Can you work these out from the drawing? Everything is in mm from the part's minimum corner. Round coordinates to 2 decimals unless told otherwise and drop trailing zeros. Order: outer loops, then holes, each group sorted by start corner. A loop starts at its lowest first (then second) coordinate and runs counter-clockwise, first axis right, second up. Notation, with made-up numbers: (12.25, -7) -> (39.25, -7) arc R34 ccw to (39.25, 30) -> close; hole circle Ø7 at (-13.75, 85). An arc over 180 degrees is marked (long way). One line per item, written item: value.
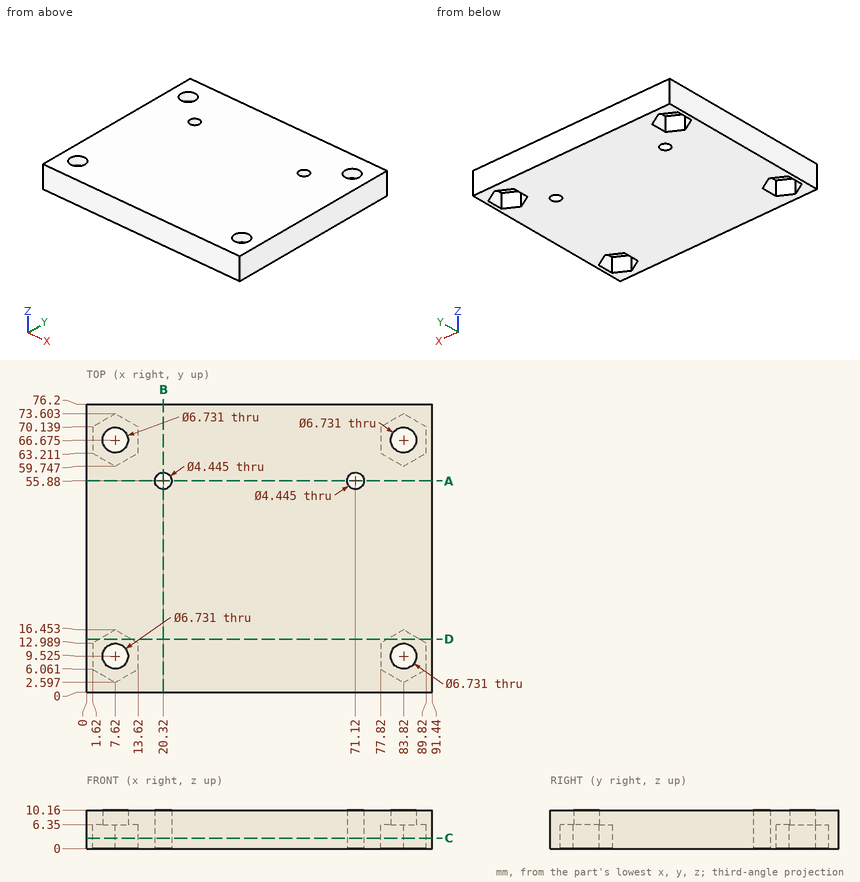
Q1. I want a section at D-D on y = 14. Write out the boundary of the cut face in (x, z), then the cut area to 3 significant figures.
Answers:
outline: (0, 0) -> (3.37, 0) -> (3.37, 6.35) -> (11.87, 6.35) -> (11.87, 0) -> (79.57, 0) -> (79.57, 6.35) -> (88.07, 6.35) -> (88.07, 0) -> (91.44, 0) -> (91.44, 10.16) -> (0, 10.16) -> close
area: 821 mm2
Q2. I want a section at A-A on y = 55.88. Write out the boundary of the cut face in (x, z).
Answers:
outline: (0, 0) -> (18.1, 0) -> (18.1, 10.16) -> (0, 10.16) -> close; (22.54, 0) -> (68.9, 0) -> (68.9, 10.16) -> (22.54, 10.16) -> close; (73.34, 0) -> (91.44, 0) -> (91.44, 10.16) -> (73.34, 10.16) -> close
Q3. I want a section at B-B on x = 20.32. Write out the boundary of the cut face in (y, z), then the cut area to 3 significant figures.
Answers:
outline: (0, 0) -> (53.66, 0) -> (53.66, 10.16) -> (0, 10.16) -> close; (58.1, 0) -> (76.2, 0) -> (76.2, 10.16) -> (58.1, 10.16) -> close
area: 729 mm2
Q4. I need wall thicknesses on line 1 along X through (y, z) = (7, 1); line 2 along X through (y, z) = (4, 4.5); line 3 along Y through (x, z) = (83.82, 8.9). Which ranges of each line are inside material? Lowest first, please.
Answers:
line 1: 0 to 1.62, 13.62 to 77.82, 89.82 to 91.44
line 2: 0 to 5.19, 10.05 to 81.39, 86.25 to 91.44
line 3: 0 to 6.16, 12.89 to 63.31, 70.04 to 76.2
Q5. I want a section at C-C on z = 2.75. Give the number of separate pieces and of enclosed holes in the cut face, then the cut area to 3 significant figures.
Answers:
separate pieces: 1
enclosed holes: 6
area: 6,440 mm2
Q6. For P1, Ø9.5, axis at x = 85, y = 67, coming from the -Z side; P2, Ø2.5, axis at x = 71.12, y = 55.88, coming from the -Z side, each with a flat end and sliding along its axis, tell me the tip position at first contact or that it passes through.
Answers:
P1: z = 6.35
P2: through
